Autodesk Inventor part; units mm, degrees
ref_plane "YZ Plane" through (0, 0, 0) normal (1, 0, 0) x (0, 1, 0)
ref_plane "XZ Plane" through (0, 0, 0) normal (0, 1, 0) x (-1, 0, 0)
ref_plane "XY Plane" through (0, 0, 0) normal (0, 0, 1) x (1, 0, 0)
sketch "Sketch2" plane through (0, 0, 0) normal (0, 0, 1) x (1, 0, 0)
  circle A0 centre (-19.05, 0) radius 3.25
  line L0 (-15.9375, 3.25) -> (19.8375, 3.25)
  arc A1 (-15.9375, 3.25) -> (-15.9375, -3.25) centre (-19.05, 0) ccw
  arc A2 (19.8375, -3.25) -> (19.8375, 3.25) centre (22.95, 0) ccw
  circle A3 centre (22.95, 0) radius 3.25
  line L1 (-31.7023, 0) -> (39.7352, 0) construction
  line L2 (-15.9375, -3.25) -> (19.8375, -3.25)
  point P0 (0, 0)
  dimension "d4" = 6.5
  dimension "d6" = 9
  dimension "d7" = 6.5
  dimension "d8" = 42
extrude "Extrusion1" add sketch "Sketch2" along normal blind 5 contours A0 | L0 A2 L2 A1 | A3
extrude "Extrusion2" add sketch "Sketch2" against normal blind 5 contours A0 | A3
equation "\"d4\" = R"
equation "\"d6\" = R1"
equation "\"d7\" = width"
equation "\"d0\" = thickness"
equation "\"d2\" = thickness"
equation "\"R\" = 6.5"
equation "\"thickness\" = 5"
equation "\"width\" = 6.5"
equation "\"R1\" = 9"
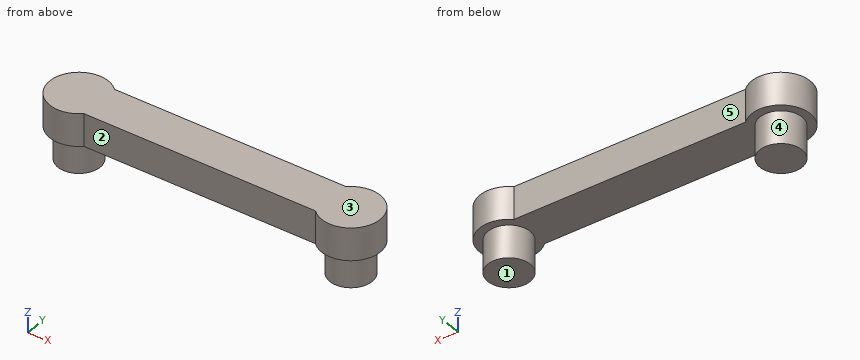
Can you work these out from the model? Positions are in its coordinate system, mm. Face numbers are marked on the shaded views. A direction names the side the tool comes from. Round coordinates to 2 decimals unless told otherwise and drop trailing zeros. Loops run counter-clockwise (first coordinate to the right, second up) from the corner with the lowest first, then second, coordinate; pieces in that order, holes last. Notation, with made-up numbers: M -10.5,42.25 L 13.5,42.25 A17 cw 13.5,74.25 Z; hole C 52,-22.5 d8. An arc over 180 degrees is marked long. Answer in a Markdown table with one row per item.
1. I'm going to push flat-ended pins straight in: pin 1 Ø1.5 at (y, z) = (3, 0.5) entering from -X; pin 2 Ø2 at (x, z) = (-4.5, 3) entering from -Y; pin 3 Ø1.5 at (x, y) = (-2.5, 2) entering from -Z. Where does each tip first touch, or does it pass through?
Established:
| item | result |
|---|---|
| pin 1 | x = -22.95 |
| pin 2 | y = -3.25 |
| pin 3 | z = 0 |
2. Thinking about a two-plate mould opening in X: for the marked faces 1 and 2, which applies, pulls with the +X half, pulls with the -X half, needs draft (parallel to the pull), parting line crosses it, or undercut?
Established:
| item | result |
|---|---|
| face 1 | needs draft |
| face 2 | undercut |
3. If we section it at D-D, the plane z = 2.5: Please give me the cut outline in (x, y), plus the area to 3 significant figures.
Established:
| item | result |
|---|---|
| outline | M -15.94,-3.25 L 19.84,-3.25 A4.5 ccw long 19.84,3.25 L -15.94,3.25 A4.5 ccw long Z |
| area | 347 mm² |
4. Please list where these lines run through material, in increasing order: line 1 (Z direction, x = -9, y = 0.25); line 2 (Y direction, x = 17, z = 1.25); line 3 (X direction, y = -2.25, z = -3.25). Write a range as from..to.
Established:
| item | result |
|---|---|
| line 1 | 0..5 |
| line 2 | -3.25..3.25 |
| line 3 | -21.4..-16.7, 20.6..25.3 |
5. On a 3-axis mill with a long thin cutter (end or side, diameter ignored), from which of +Z, -Z, +X, -X, +Y, -Y can I reach the whole of each face in a straight line? I mean the marked faces 3, 4 and 5. Say none if no direction works.
Established:
| item | result |
|---|---|
| face 3 | +Z, +X, -X, +Y, -Y |
| face 4 | -Z |
| face 5 | +Z, -Z, +Y |
6. If we section it at B-B, the plane y = 0: Please give me the cut outline in (x, z), plus the area to 3 significant figures.
Established:
| item | result |
|---|---|
| outline | M -23.55,0 L -22.3,0 L -22.3,-5 L -15.8,-5 L -15.8,0 L 19.7,0 L 19.7,-5 L 26.2,-5 L 26.2,0 L 27.45,0 L 27.45,5 L -23.55,5 Z |
| area | 320 mm² |
7. If we section it at A-A, the plane z = -2: Please give me the cut outline in (x, y).
Established:
| item | result |
|---|---|
| outline | C -19.05,0 d6.5; C 22.95,0 d6.5 |
8. If we section it at C-C, the plane x = -19.05: Please give me the cut outline in (y, z).
Established:
| item | result |
|---|---|
| outline | M -4.5,0 L -3.25,0 L -3.25,-5 L 3.25,-5 L 3.25,0 L 4.5,0 L 4.5,5 L -4.5,5 Z |
